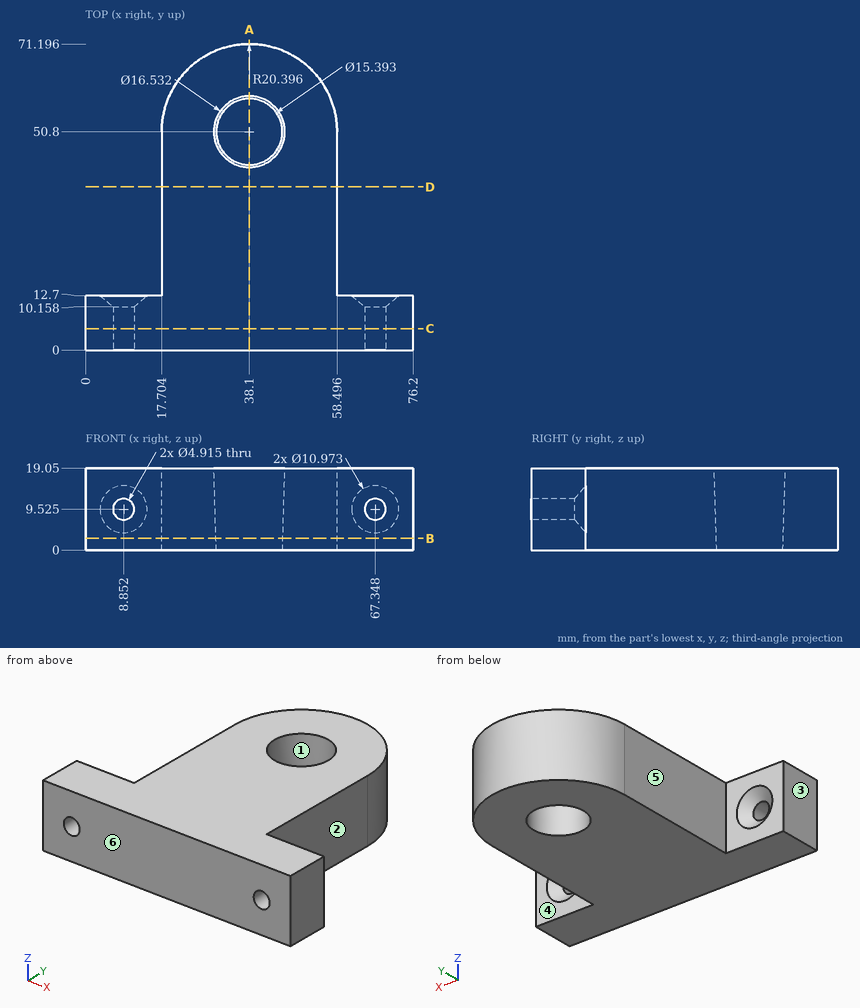
Design review of the part shown in the three views and the two pictorial views. Dimensions are in mm from the part's minimum x, y and z. A direction names the side the tool comes from. Coordinates: 2 decimals unless noted, no trailing zeros. Order: outer loops, then holes, each group sorted by start corner. A loop starts at its lowest first (then second) coordinate and runs counter-clockwise, first axis right, second up.
Item 1: For pin 1 Ø5.5 at (x, z) = (63.5, 12) entering from +Y; pin 2 Ø4 at (y, z) = (37.5, 16.5) entering from -X; pin 3 Ø2 at (y, z) = (22.5, 14) entering from +X, all flat-tipped, find the tip position at first contact; note any pin that passes through.
Item 2: The part is to be moulded in two halves that separate along X. For the marked faces 1, 2 and 3, say which applies: pulls with the +X half, pulls with the -X half, needs draft (parallel to the pull), parting line crosses it, or undercut.
Item 3: Take a section at A-A, the plane x = 38.1. Write out the cut boundary in (y, z), then the cut area to 3 significant figures.
Item 4: Take a section at D-D, the plane y = 38. Write out the cut boundary in (x, z).
Item 5: Take a section at B-B, the plane z = 2.75. Write out the cut boundary in (x, y).
Item 6: Take a section at C-C, the plane y = 5. Count the separate pieces of the cut face and the enclosed holes in it, then the cut area to 3 significant figures.
Item 7: For the marked faces 4, 5 and 6, list the 3-axis set-ups (+Z, -Z, +X, -X, +Y, -Y) from which the entire face can be reached by the end or side of a thin tool; tool diameter is ignored.
Item 8: For line 1 (X direction, y = 31, z = 16.75); line 2 (Y direction, x = 59, z = 11.5); line 3 (X direction, y = 48, z = 11) (1 decimal), list the stretches that pass through material, from the lowest coordinate up.
The answers:
1. pin 1: stops at y = 12.7
1. pin 2: stops at x = 17.7
1. pin 3: stops at x = 58.5
2. face 1: undercut
2. face 2: pulls with the +X half
2. face 3: pulls with the -X half
3. outline: (0, 0) - (43.1, 0) - (42.53, 19.05) - (0, 19.05) - close; (58.5, 0) - (71.2, 0) - (71.2, 19.05) - (59.07, 19.05) - close
3. area: 1,050 mm2
4. outline: (17.7, 0) - (58.5, 0) - (58.5, 19.05) - (17.7, 19.05) - close
5. outline: (0, 0) - (76.2, 0) - (76.2, 12.7) - (58.5, 12.7) - (58.5, 50.8) arc R20.4 ccw to (17.7, 50.8) - (17.7, 12.7) - (0, 12.7) - close; hole circle Ø15.56 at (38.1, 50.8)
6. separate pieces: 1
6. enclosed holes: 2
6. area: 1,410 mm2
7. face 4: +Z, -Z, +X, +Y
7. face 5: +Z, -Z, -X, +Y
7. face 6: +Z, -Z, +X, -X, -Y
8. line 1: x = 17.7 to 58.5
8. line 2: y = 0 to 12.7
8. line 3: x = 17.7 to 30.6, 45.6 to 58.5
